Design review of the part built by this model. Coordinates are the model's own, in mm. A direction names the side the tool comes from. Give positions to 0.01 mm unless a question says otherwise; leave off trailing zeros. Write each loop counter-clockwise with the first axis right and the second up, starting at its lowest first coordinate (ties: lowest second). Pieces come first, ordered by that corner, then holes.
```python
from build123d import *

# Parameters (mm, degrees)
ESQUISSE1_W                  = 540
ESQUISSE1_H                  = 39
BOSS_EXTRU_1_DEPTH           = 10
CONG_1_R                     = 15
ESQUISSE3_W                  = 10
ESQUISSE3_H                  = 39
BOSS_EXTRU_2_DEPTH           = 42
ESQUISSE4_W                  = 540
ESQUISSE4_H                  = 39
BOSS_EXTRU_3_DEPTH           = 10
CONG_2_R                     = 15
ENL_V_MAT_EXTRU_2_DEPTH      = 278.712531226
ENL_V_MAT_EXTRU_2_DEPTH_BACK = 278.712531226
ESQUISSE5_R                  = 4
ESQUISSE6_R                  = 1
BOSS_EXTRU_4_DEPTH           = 10
ENL_V_MAT_EXTRU_3_DEPTH      = 280.758824704
ENL_V_MAT_EXTRU_3_DEPTH_BACK = 280.758824704
ESQUISSE7_W                  = 440
ESQUISSE7_H                  = 10
ENL_V_MAT_EXTRU_4_DEPTH      = 277.53978014
ENL_V_MAT_EXTRU_4_DEPTH_BACK = 277.53978014
ESQUISSE13_W                 = 440
ESQUISSE13_H                 = 39
BOSS_EXTRU_6_REACH           = 496.787
ESQUISSE14_R                 = 4


with BuildPart() as part:
    # Esquisse1 → Boss.-Extru.1 (new body)
    with BuildSketch(Plane(origin=(0, 0, 0), x_dir=(1, 0, 0), z_dir=(0, 1, 0))):
        Rectangle(ESQUISSE1_W, ESQUISSE1_H)
    extrude(amount=BOSS_EXTRU_1_DEPTH)

    # Cong_1
    cong_1_edges = [part.edges().sort_by_distance(p)[0] for p in [
        (270, 5, 19.5),
        (-270, 5, 19.5),
        (-270, 5, -19.5),
        (270, 5, -19.5),
    ]]
    fillet(cong_1_edges, radius=CONG_1_R)

    # Esquisse3 → Boss.-Extru.2 (add)
    with BuildSketch(Plane(origin=(0, 10, 0), x_dir=(1, 0, 0), z_dir=(0, 1, 0))):
        with Locations((-225, 0)):
            Rectangle(ESQUISSE3_W, ESQUISSE3_H)
        with Locations((225, 0)):
            Rectangle(ESQUISSE3_W, ESQUISSE3_H)
    extrude(amount=BOSS_EXTRU_2_DEPTH)

    # Esquisse4 → Boss.-Extru.3 (add)
    with BuildSketch(Plane(origin=(0, 52, 0), x_dir=(1, 0, 0), z_dir=(0, 1, 0))):
        Rectangle(ESQUISSE4_W, ESQUISSE4_H)
    extrude(amount=BOSS_EXTRU_3_DEPTH)

    # Cong_2
    cong_2_edges = [part.edges().sort_by_distance(p)[0] for p in [
        (-270, 57, -19.5),
        (-270, 57, 19.5),
        (270, 57, 19.5),
        (270, 57, -19.5),
    ]]
    fillet(cong_2_edges, radius=CONG_2_R)

    # Esquisse5 → Enl_v. mat.-Extru.2 (cut, two sides: drawn at the far end of the back side and taken through both)
    with BuildSketch(Plane(origin=(0, 62, 0), x_dir=(1, 0, 0), z_dir=(0, 1, 0)).offset(-ENL_V_MAT_EXTRU_2_DEPTH_BACK)):
        with Locations(Location((249, 0, 0), (0, 0, 270))):
            Circle(ESQUISSE5_R)
        with Locations(Location((-249, 0, 0), (0, 0, 270))):
            Circle(ESQUISSE5_R)
    extrude(amount=ENL_V_MAT_EXTRU_2_DEPTH + ENL_V_MAT_EXTRU_2_DEPTH_BACK, mode=Mode.SUBTRACT)

    # Esquisse6 → Boss.-Extru.4 (add)
    with BuildSketch(Plane.XY.offset(19.5)):
        with Locations(Location((-235, 57, 0), (0, 0, 180))):
            Circle(ESQUISSE6_R)
        with Locations(Location((-235, 5, 0), (0, 0, 180))):
            Circle(ESQUISSE6_R)
        with Locations(Location((235, 5, 0), (0, 0, 180))):
            Circle(ESQUISSE6_R)
        with Locations(Location((235, 57, 0), (0, 0, 180))):
            Circle(ESQUISSE6_R)
    extrude(amount=BOSS_EXTRU_4_DEPTH)

    # Esquisse7 → Enl_v. mat.-Extru.3 (cut, two sides: drawn at the far end of the back side and taken through both)
    with BuildSketch(Plane.XY.offset(19.5).offset(-ENL_V_MAT_EXTRU_3_DEPTH_BACK)):
        with Locations((0, 57)):
            Rectangle(ESQUISSE7_W, ESQUISSE7_H)
    extrude(amount=ENL_V_MAT_EXTRU_3_DEPTH + ENL_V_MAT_EXTRU_3_DEPTH_BACK, mode=Mode.SUBTRACT)

    # Esquisse13 → Enl_v. mat.-Extru.4 (cut, two sides: drawn at the far end of the back side and taken through both)
    with BuildSketch(Plane(origin=(0, 10, 0), x_dir=(1, 0, 0), z_dir=(0, 1, 0)).offset(-ENL_V_MAT_EXTRU_4_DEPTH_BACK)):
        Rectangle(ESQUISSE13_W, ESQUISSE13_H)
    extrude(amount=ENL_V_MAT_EXTRU_4_DEPTH + ENL_V_MAT_EXTRU_4_DEPTH_BACK, mode=Mode.SUBTRACT)


with BuildPart() as enl_v_mat_extru_4_piece_1:
    # of the separate pieces the step leaves, piece 1, a body of its own (enl_v_mat_extru_4_pieces)
    add(part.part.solids().sort_by_distance((220, 0, -19.5))[0])

    # Esquisse14 → Boss.-Extru.6 (add, up to next)
    with BuildSketch(Plane(origin=(-220, 0, 0), x_dir=(0, 0, -1), z_dir=(1, 0, 0)), mode=Mode.PRIVATE) as boss_extru_6_sk1:
        with Locations((0, 52)):
            Circle(ESQUISSE14_R)
    boss_extru_6_tool1 = extrude(boss_extru_6_sk1.sketch, amount=BOSS_EXTRU_6_REACH, mode=Mode.PRIVATE) - enl_v_mat_extru_4_piece_1.part
    # Esquisse14 → Boss.-Extru.6 (add, up to next)
    with BuildSketch(Plane(origin=(-220, 0, 0), x_dir=(0, 0, -1), z_dir=(1, 0, 0)), mode=Mode.PRIVATE) as boss_extru_6_sk2:
        with Locations(Location((0, 10, 0), (0, 0, 180))):
            Circle(ESQUISSE14_R)
    boss_extru_6_tool2 = extrude(boss_extru_6_sk2.sketch, amount=BOSS_EXTRU_6_REACH, mode=Mode.PRIVATE) - enl_v_mat_extru_4_piece_1.part


with BuildPart() as enl_v_mat_extru_4_piece_2:
    # of the separate pieces the step leaves, piece 2, a body of its own (enl_v_mat_extru_4_pieces)
    add(part.part.solids().sort_by_distance((-255, 52, -19.5))[0])


with BuildPart() as enl_v_mat_extru_4_piece_1_1:
    add(enl_v_mat_extru_4_piece_1.part)

    add(enl_v_mat_extru_4_piece_2.part)  # Boss.-Extru.6 merges Enl_v. mat.-Extru.4 piece 2
    add(boss_extru_6_tool1.solids().sort_by_distance((-220, 52, 0))[0])
    add(boss_extru_6_tool2.solids().sort_by_distance((-220, 10, 0))[0])


solid = enl_v_mat_extru_4_piece_1_1.part
```
(1) Clearance check with flat-ended pins moving along their axes: P1, Ø19.5, axis at y = 37, z = 0, coming from the +X side; P2, Ø5, axis at x = -60, z = 1, coming from the +Y side; P3, Ø2, axis at y = 18, z = -6, coming from the -X side; P4, Ø4, axis at x = 213, z = 7.5, coming from the +Y side. State where each tip first meets the part, or that it passes through.
Resolved:
P1: stops at x = 230
P2: stops at y = 56
P3: stops at x = -230
P4: passes through
(2) Consider section D-D, the plane z = 14. Give the boundary of the cut face in (x, y).
Resolved:
outline: (-266.61, 0) - (-220, 0) - (-220, 62) - (-266.61, 62) - (-266.61, 52) - (-230, 52) - (-230, 10) - (-266.61, 10) - close; (220, 0) - (266.61, 0) - (266.61, 10) - (230, 10) - (230, 52) - (266.61, 52) - (266.61, 62) - (220, 62) - close
(3) Consider section C-C, the plane x = 133.5. Give the boundary of the cut face in (y, z), then the cut area to 3 significant figures.
Resolved:
outline: circle Ø8 at (10, 0); circle Ø8 at (52, 0)
area: 101 mm2
(4) Consider section B-B, the plane z = -11. Give the boundary of the cut face in (x, y), then the cut area to 3 significant figures.
Resolved:
outline: (-268.52, 0) - (-220, 0) - (-220, 62) - (-268.52, 62) - (-268.52, 52) - (-230, 52) - (-230, 10) - (-268.52, 10) - close; (220, 0) - (268.52, 0) - (268.52, 10) - (230, 10) - (230, 52) - (268.52, 52) - (268.52, 62) - (220, 62) - close
area: 2,780 mm2
(5) Consider section A-A, the plane y = 21. Give the boundary of the cut face in (x, z).
Resolved:
outline: (-230, -19.5) - (-220, -19.5) - (-220, 19.5) - (-230, 19.5) - close; (220, -19.5) - (230, -19.5) - (230, 19.5) - (220, 19.5) - close
(6) Tool access review of faces 1 (the face through (-230, 31, 0)), 2 (the face through (265.49, 57.07, -15.22)): name each direction out of +Z, -Z, +X, -X, +Y, -Y from which nothing blocks a thin tool from reaching the whole face with its end or side.
Resolved:
face 1: +Z, -Z, -X
face 2: -Z, +X, +Y, -Y
(7) To check wall thickness, follow L1, parallel to X at y = 7, z = 0; L2, parallel to X at y = 4.25, z = 0; L3, parallel to Z at x = -249, y = 56. State the ranges of each line that lie inside material, in increasing order.
Resolved:
L1: x = -270 to -253, -245 to 245, 253 to 270
L2: x = -270 to -253, -245 to -220, 220 to 245, 253 to 270
L3: z = -19.5 to -4, 4 to 19.5
(8) Mouldability with a two-part tool opening along Y and no side actions: class faces 3 (the face through (-265.72, 57.07, -14.99)), 4 (the face through (249.7, 52, 4.1)), 5 (the face through (249.7, 10, 4.1)), 6 (the face through (244.6, 0, -0.3)) as pulls with the +Y half, pulls with the -Y half, needs draft (parallel to the pull), parting line crosses it, or undercut.
Resolved:
face 3: needs draft
face 4: undercut
face 5: undercut
face 6: pulls with the -Y half
